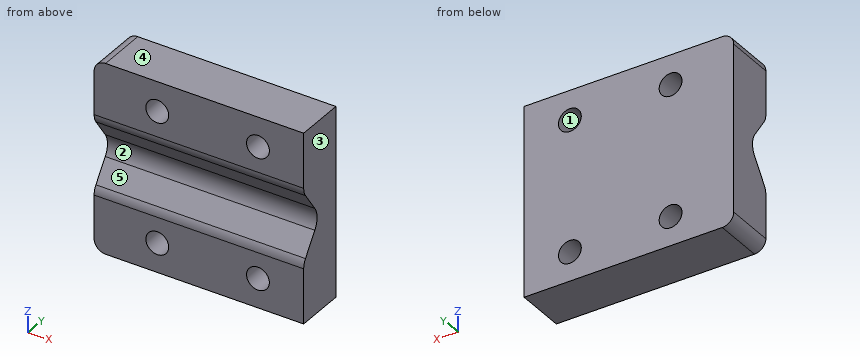
from build123d import *

# Parameters (mm, degrees)
SKETCH6_W          = 55.097235346
SKETCH6_H          = 50
MAIN_BODY_DEPTH    = 13
MAIN_HOLE_DEPTH    = 56.097235346
EXTERIOR_FILLET_R  = 3
SKETCH9_R          = 3
BOLT_HOLES_DEPTH   = 14
TOP_HOLE_FILLET_R  = 5
SIDE_HOLE_FILLET_R = 4


with BuildPart() as part:
    # Sketch6 → Main Body (new body)
    with BuildSketch(Plane(origin=(0, 68, 0), x_dir=(1, 0, 0), z_dir=(0, 1, 0))):
        with Locations((-0.048617673, 0)):
            Rectangle(SKETCH6_W, SKETCH6_H)
    extrude(amount=MAIN_BODY_DEPTH)

    # Sketch7 → Main Hole (cut, through all)
    with BuildSketch(Plane(origin=(27.5, 0, 0), x_dir=(0, 0, -1), z_dir=(1, 0, 0))):
        Polygon((0, 74.5), (-9.282962044, 68), (0, 61.5), (9.282962044, 68), align=None)
    extrude(amount=-MAIN_HOLE_DEPTH, mode=Mode.SUBTRACT)

    # Exterior Fillet
    exterior_fillet_edges = [part.edges().sort_by_distance(p)[0] for p in [
        (-27.597235346, 74.5, 25),
        (-27.597235346, 74.5, -25),
    ]]
    fillet(exterior_fillet_edges, radius=EXTERIOR_FILLET_R)

    # Sketch9 → Bolt Holes (cut, through all)
    with BuildSketch(Plane(origin=(0, 81, 0), x_dir=(1, 0, 0), z_dir=(0, 1, 0))):
        with Locations((15.473743703, -17.201232435)):
            Circle(SKETCH9_R)
        with Locations((-11, -17.201232435)):
            Circle(SKETCH9_R)
        with Locations((15.473743703, 17.324336932)):
            Circle(SKETCH9_R)
        with Locations((-11, 17.324336932)):
            Circle(SKETCH9_R)
    extrude(amount=-BOLT_HOLES_DEPTH, mode=Mode.SUBTRACT)

    # Top Hole Fillet
    top_hole_fillet_edges = [part.edges().sort_by_distance(p)[0] for p in [
        (-0.048617673, 74.5, 0),
    ]]
    fillet(top_hole_fillet_edges, radius=TOP_HOLE_FILLET_R)

    # Side Hole Fillet
    side_hole_fillet_edges = [part.edges().sort_by_distance(p)[0] for p in [
        (-0.048617673, 68, -9.282962044),
        (-0.048617673, 68, 9.282962044),
    ]]
    fillet(side_hole_fillet_edges, radius=SIDE_HOLE_FILLET_R)


solid = part.part
Geometry check sheet. Reference: the model listing, model coordinates, mm. Face numbers are marked on the shaded views. A direction names the side the tool comes from. Give positions to 0.01 mm unless a question says otherwise; leave off trailing zeros. Order: outer loops, then holes, each group sorted by start corner. A loop starts at its lowest first (then second) coordinate and runs counter-clockwise, first axis right, second up. Notation, with made-up numbers: (59.25, -24) - (86.25, -24) arc R29 cw to (86.25, -2) - close; hole circle Ø6 at (-21, 35.25). An arc over 180 degrees is marked (long way). Use one line per item in the form item = value.
1) Sectioned sample at A-A (y = 70.25). Record the boundary of the cut face in (x, z).
Working result:
outline = (-27.6, -22) arc R3 ccw to (-24.6, -25) - (27.5, -25) - (27.5, -6.07) - (-27.6, -6.07) - close; (-27.6, 6.07) - (27.5, 6.07) - (27.5, 25) - (-24.6, 25) arc R3 ccw to (-27.6, 22) - close; hole circle Ø6 at (-11, -17.32); hole circle Ø6 at (-11, 17.2); hole circle Ø6 at (15.47, -17.32); hole circle Ø6 at (15.47, 17.2)
2) Access from +Z, -Z, +X, -X, +Y, -Y to the whole of each face (thin tool, end or side, straight path). Record for the marked faces 4 and 5.
Working result:
face_4 = +Z, +X, -X, +Y, -Y
face_5 = +X, -X, -Y
3) Depth check by flat-ended pin: pin 1 Ø5.5 at (x, z) = (15.47, -17.32) entering from +Y. Enter the tip coordinate at first touch or a pass-through.
Working result:
pin_1 = through
4) Material ranges on probe 1 along Z at (x, y) = (-11, 77); probe 2 along Z at (x, y) = (16.5, 69.5); probe 3 along Z at (x, y) = (13, 78.5), recorded low to high. Write a range as from..to.
Working result:
probe_1 = -25..-20.32, -14.32..14.2, 20.2..25
probe_2 = -25..-20.14, -14.51..-7.14, 7.14..14.38, 20.02..25
probe_3 = -25..-19.02, -15.63..15.5, 18.9..25
5) Sectioned sample at D-D (y = 75). Record the boundary of the cut face in (x, z), and give its area (3 significant figures).
Working result:
outline = (-27.6, -22) arc R3 ccw to (-24.6, -25) - (27.5, -25) - (27.5, 25) - (-24.6, 25) arc R3 ccw to (-27.6, 22) - close; hole circle Ø6 at (-11, -17.32); hole circle Ø6 at (-11, 17.2); hole circle Ø6 at (15.47, -17.32); hole circle Ø6 at (15.47, 17.2)
area = 2,640 mm^2
6) Sectioned sample at C-C (z = 19.5). Record the boundary of the cut face in (x, y).
Working result:
outline = (-27.6, 68) - (-12.93, 68) - (-12.93, 81) - (-27.6, 81) - close; (-9.07, 68) - (13.55, 68) - (13.55, 81) - (-9.07, 81) - close; (17.4, 68) - (27.5, 68) - (27.5, 81) - (17.4, 81) - close
7) Draft check along X on the marked faces 1, 2 and 3. Enter one of: released by +X, released by -X, zero draft, split by the parting line, or undercut.
Working result:
face_1 = undercut
face_2 = zero draft
face_3 = released by +X
8) Sectioned sample at B-B (x = -11). Record the boundary of the cut face in (y, z).
Working result:
outline = (68, -25) - (81, -25) - (81, -20.32) - (68, -20.32) - close; (68, -14.32) - (81, -14.32) - (81, 14.2) - (68, 14.2) - (68, 10.54) arc R4 ccw to (68.72, 8.25) - (72.49, 2.87) arc R5 cw to (72.49, -2.87) - (68.72, -8.25) arc R4 ccw to (68, -10.54) - close; (68, 20.2) - (81, 20.2) - (81, 25) - (68, 25) - close
